from build123d import *

# Parameters (mm, degrees)
CHAPAINFERIOR_DEPTH = 4


with BuildPart() as part:
    # Chapa inferior → ChapaInferior (new, symmetric)
    with BuildSketch(Plane(origin=(0, 0, 0), x_dir=(1, 0, 0), z_dir=(0, 1, 0))):
        with BuildLine():
            Line((-160, 300), (160, 300))
            ThreePointArc((160, 300), (230.710678119, 270.710678119), (260, 200))
            Line((260, 200), (260, -200))
            ThreePointArc((260, -200), (230.710678119, -270.710678119), (160, -300))
            Line((160, -300), (-160, -300))
            ThreePointArc((-160, -300), (-230.710678119, -270.710678119), (-260, -200))
            Line((-260, -200), (-260, 200))
            ThreePointArc((-260, 200), (-230.710678119, 270.710678119), (-160, 300))
        make_face()
    extrude(amount=CHAPAINFERIOR_DEPTH, both=True)


solid = part.part
The model under review builds one solid part; all positions refer to its coordinate system, in mm. Round coordinates to 2 decimals unless told otherwise and drop trailing zeros. Loops run counter-clockwise (first coordinate to the right, second up) from the corner with the lowest first, then second, coordinate; pieces in that order, holes last. Notation, with made-up numbers: M 74,81.25 L 80,81.25 A33 cw 80,116.25 Z; hole C 43.5,-33 d4. An arc over 180 degrees is marked long. Answer as a JSON object with one key per item and string values.
Item 1: The part is to be moulded in two halves that separate along Z. For faces 1 (the face through (4, 4, -4)), 2 (the face through (-229.929, 0.056, 271.484)), 3 (the face through (-231.484, 0.056, -269.929)), say which applies: +Z half, -Z half, draft (parallel to the pull), parting line (faces both ways), or undercut.
Check sheet entries:
{"face 1": "draft", "face 2": "+Z half", "face 3": "-Z half"}
Item 2: We need section B-B, the plane x = -212. State the section outline as (y, z) points.
Check sheet entries:
{"outline": "M -4,-285.42 L 4,-285.42 L 4,285.42 L -4,285.42 Z"}
Item 3: We need section A-A, the plane y = -2. State the section outline as (x, z) points, and give its area (3 significant figures).
Check sheet entries:
{"outline": "M -260,-200 A100 ccw -160,-300 L 160,-300 A100 ccw 260,-200 L 260,200 A100 ccw 160,300 L -160,300 A100 ccw -260,200 Z", "area": "303,000 mm2"}
Item 4: For line 1 along Z through (x, y) = (-161.5, 0.75); line 2 along X through (y, z) = (-3, -205); line 3 along Z through (x, y) = (199, 2.75), list the stretches that pass through material, from the lowest coordinate up.
Check sheet entries:
{"line 1": "-299.99 to 299.99", "line 2": "-259.87 to 259.87", "line 3": "-292.08 to 292.08"}
Item 5: Clearance check with a flat-ended pin moving along its axis: P1, Ø1.5, axis at x = -171, y = -1.5, coming from the -Z side. State where the tip first meets the part, or that it passes through.
Check sheet entries:
{"P1": "z = -299.47"}
